For this review, take the finished solid that the model builds, in its own axes (mm). A direction names the side the tool comes from. Coordinates: 2 decimals unless noted, no trailing zeros. Write each loop counter-clockwise with the first axis right and the second up, starting at its lowest first coordinate (ties: lowest second). Pieces come first, ordered by that corner, then holes.
1) We need section B-B on z = 20. Write out the cut boundary in (x, y), then the cut area to 3 significant figures.
2) To check wall thickness, follow line 1 along Z through (x, y) = (-32.75, 25.75); line 2 along Z through (x, y) = (-36.5, 24.25); line 3 along Y through (x, z) = (-23.5, 15). State the ranges of each line that lie inside material, in increasing order.
3) Insertion check: P1, Ø8, axis at x = 4.5, y = 5.5, coming from the +Z side; P2, Ø6, axis at x = -29.5, z = 36, coming from the +Y side; P3, Ø20, axis at x = -4.5, z = 27.5, coming from the +Y side. Each pin has a flat end and moves straight along its axis. Give the tip position at first contact, or say it passes through.
4) For faces 4 (the face through (2.28, 5.07, 37.35)), 5 (the face through (-16, 10, 11)), 6 (the face through (-32, 23, 8.5)), list the 3-axis set-ups (+Z, -Z, +X, -X, +Y, -Y) from which the entire face can be reached by the end or side of a thin tool; tool diameter is ignored.
5) Mouldability with a two-part tool opening along Z and no side actions: class faces 1 (the face through (-2, 5, 40)), 2 (the face through (16.06, 5.07, 37.783)), 3 (the face through (-17, 7, 0)) as pulls with the +Z half, pulls with the -Z half, needs draft (parallel to the pull), parting line crosses it, or undercut.
6) We need section C-C on x = -35. Write out the cut boundary in (y, z), then the cut area to 3 significant figures.
7) We need section A-A on y = 21. Write out the cut boundary in (x, z), then the cut area to 3 significant figures.
8) We need section D-D on x = 0. Write out the cut boundary in (y, z).
from build123d import *

# Parameters (mm, degrees)
F1_DEPTH = 40
F0_W     = 16.7
F0_H     = 20
F2_DEPTH = 80
F3_R     = 2
F3_R_2   = 17.5
F4_DEPTH = 10.001
F5_R     = 2.5
F6_DEPTH = 60.001
F7_W     = 16.7
F7_H     = 10
F8_DEPTH = 40


with BuildPart() as f1:
    # F0 (on Top) → F1 (new body)
    with BuildSketch(Plane.XY):
        Polygon((-15.8, 10), (-20, 10), (-20, 0), (20, 0), (20, 10), (15.8, 10), align=None)
        Polygon((-23.3, 10), (-40, 10), (-40, 0), (-20, 0), (-20, 10), align=None)
    extrude(amount=F1_DEPTH)

    # F0 (on Top) → F2 (join)
    with BuildSketch(Plane.XY):
        with Locations((-31.65, 20)):
            Rectangle(F0_W, F0_H)
    extrude(amount=F2_DEPTH)

    # F3 (on face) → F4 (cut, through all)
    with BuildSketch(Plane(origin=(0, 10, 0), x_dir=(-1, 0, 0), z_dir=(0, 1, 0))):
        with Locations((-15.8, 4.2)):
            Circle(F3_R)
        with Locations((-15.8, 35.8)):
            Circle(F3_R)
        with Locations((15.8, 35.8)):
            Circle(F3_R)
        with Locations((15.8, 4.2)):
            Circle(F3_R)
        with Locations((0, 20)):
            Circle(F3_R_2)
    extrude(amount=-F4_DEPTH, mode=Mode.SUBTRACT)

    # F5 (on face) → F6 (cut, through all)
    with BuildSketch(Plane(origin=(-40, 0, 0), x_dir=(0, -1, 0), z_dir=(-1, 0, 0))):
        with Locations((-25.75, 75.75)):
            Circle(F5_R)
        with BuildLine():
            Line((-30, 80), (-30, 75.75))
            ThreePointArc((-30, 75.75), (-28.75520382, 78.75520382), (-25.75, 80))
            Line((-25.75, 80), (-30, 80))
        make_face()
        with BuildLine():
            Line((-20, 71.5), (-25.75, 71.5))
            ThreePointArc((-25.75, 71.5), (-28.75520382, 72.74479618), (-30, 75.75))
            Line((-30, 75.75), (-30, 4.2499999975))
            ThreePointArc((-30, 4.2499999975), (-28.7552038209, 7.2552038191), (-25.75, 8.5))
            Line((-25.75, 8.5), (-20, 8.5))
            Line((-20, 8.5), (-20, 71.5))
        make_face()
        with BuildLine():
            ThreePointArc((-25.75, 0), (-28.7552038191, 1.2447961791), (-30, 4.2499999975))
            Line((-30, 4.2499999975), (-30, 0))
            Line((-30, 0), (-25.75, 0))
        make_face()
        with Locations((-25.75, 4.25)):
            Circle(F5_R)
    extrude(amount=-F6_DEPTH, mode=Mode.SUBTRACT)

    # F7 (on face) → F8 (join, through all)
    with BuildSketch(Plane.XY.offset(40)):
        with Locations((-31.65, 5)):
            Rectangle(F7_W, F7_H)
    extrude(amount=F8_DEPTH)


solid = f1.part
Result:
1. outline: (-40, 0) - (-17.5, 0) - (-17.5, 10) - (-23.3, 10) - (-23.3, 20) - (-40, 20) - close; (17.5, 0) - (20, 0) - (20, 10) - (17.5, 10) - close
1. area: 417 mm2
2. line 1: z = 0 to 1.75, 6.75 to 8.5, 71.5 to 73.25, 78.25 to 80
2. line 2: z = 0 to 2.25, 6.25 to 8.5, 71.5 to 73.75, 77.75 to 80
2. line 3: y = 0 to 20
3. P1: stops at z = 40
3. P2: stops at y = 20
3. P3: stops at y = 10
4. face 4: +Y, -Y
4. face 5: +Z, -Z, +X, +Y
4. face 6: +X, -X, +Y
5. face 1: pulls with the +Z half
5. face 2: undercut
5. face 3: pulls with the -Z half
6. outline: (0, 0) - (25.75, 0) arc R4.25 ccw to (25.75, 8.5) - (20, 8.5) - (20, 71.5) - (25.75, 71.5) arc R4.25 ccw to (25.75, 80) - (0, 80) - close; hole circle Ø5 at (25.75, 4.25); hole circle Ø5 at (25.75, 75.75)
6. area: 1,720 mm2
7. outline: (-40, 0) - (-23.3, 0) - (-23.3, 8.5) - (-40, 8.5) - close; (-40, 71.5) - (-23.3, 71.5) - (-23.3, 80) - (-40, 80) - close
7. area: 284 mm2
8. outline: (0, 0) - (10, 0) - (10, 2.5) - (0, 2.5) - close; (0, 37.5) - (10, 37.5) - (10, 40) - (0, 40) - close
